The model under review builds one solid part; all positions refer to its coordinate system, in mm. Face numbers are marked on the shaded views. A direction names the side the tool comes from. Round coordinates to 2 decimals unless told otherwise and drop trailing zeros. Write each loop counter-clockwise with the first axis right and the second up, starting at its lowest first coordinate (ties: lowest second). Pieces come first, ordered by that corner, then holes. Notation, with made-up numbers: (38, 88) - (68, 88) arc R18 ccw to (68, 119) - close; hole circle Ø1 at (-17, 64.5). An arc over 180 degrees is marked (long way). Return JSON: item names as keys, results as strings.
from build123d import *

# Parameters (mm, degrees)
BOSS_EXTRUDE1_DEPTH = 40
SKETCH2_R           = 12.7
CUT_EXTRUDE2_DEPTH  = 40


with BuildPart() as part:
    # Sketch1 → Boss-Extrude1 (new body)
    with BuildSketch(Plane.XY):
        with BuildLine():
            Line((133.254134777, 0), (133.254134777, 8))
            Line((133.254134777, 8), (91.254134777, 8))
            ThreePointArc((91.254134777, 8), (33.254134777, 58.549124673), (-24.745865223, 8))
            Line((-24.745865223, 8), (-66.745865223, 8))
            Line((-66.745865223, 8), (-66.745865223, 0))
            Line((-66.745865223, 0), (-16.745865223, 0))
            ThreePointArc((-16.745865223, 0), (33.254134777, 50), (83.254134777, 0))
            Line((83.254134777, 0), (133.254134777, 0))
        make_face()
    extrude(amount=BOSS_EXTRUDE1_DEPTH)

    # Sketch2 → Cut-Extrude2 (cut)
    with BuildSketch(Plane(origin=(0, 8, 0), x_dir=(1, 0, 0), z_dir=(0, 1, 0))):
        with Locations(Location((-46.745865223, -20, 0), (0, 0, 180))):
            Circle(SKETCH2_R)
        with Locations(Location((113.254134777, -20, 0), (0, 0, 180))):
            Circle(SKETCH2_R)
    extrude(amount=-CUT_EXTRUDE2_DEPTH, mode=Mode.SUBTRACT)


solid = part.part
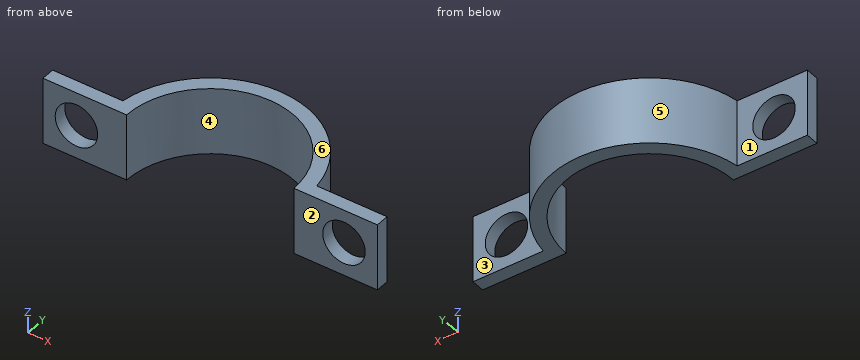
(1) Add section D-D (z = 9). Write out the cut boundary in (x, y), plus the area to 3 significant figures.
Filled in:
{"outline": "(-66.75, 0) - (-53.09, 0) - (-53.09, 8) - (-66.75, 8) - close; (-40.4, 0) - (-16.75, 0) arc R50 cw to (83.25, 0) - (106.91, 0) - (106.91, 8) - (91.25, 8) arc R58.55 ccw to (-24.75, 8) - (-40.4, 8) - close; (119.6, 0) - (133.25, 0) - (133.25, 8) - (119.6, 8) - close", "area": "1,920 mm2"}
(2) Add section B-B (y = 22.5). Write out the cut boundary in (x, z).
Filled in:
{"outline": "(-20.8, 0) - (-11.4, 0) - (-11.4, 40) - (-20.8, 40) - close; (77.91, 0) - (87.31, 0) - (87.31, 40) - (77.91, 40) - close"}
(3) Add section C-C (x = 103.5). Write out the cut boundary in (y, z), plus the area to 3 significant figures.
Filled in:
{"outline": "(0, 0) - (8, 0) - (8, 11.87) - (0, 11.87) - close; (0, 28.13) - (8, 28.13) - (8, 40) - (0, 40) - close", "area": "190 mm2"}
(4) Clearance check with flat-ended pins moving along their axes: pin 1 Ø5 at (y, z) = (21.5, 18) entering from +X; pin 2 Ø23 at (x, z) = (113.25, 20) entering from +Y; pin 3 Ø1.5 at (y, z) = (15, 35) entering from -X; pin 4 Ø20 at (x, z) = (-49, 10.5) entering from +Y. State where each tip first meets the part, or that it passes through.
Filled in:
{"pin 1": "stops at x = 88.63", "pin 2": "passes through", "pin 3": "stops at x = -23.53", "pin 4": "stops at y = 8"}
(5) For the marked faces 1, 2 and 3, list the 3-axis set-ups (+Z, -Z, +X, -X, +Y, -Y) from which the entire face can be reached by the end or side of a thin tool; tool diameter is ignored.
Filled in:
{"face 1": "+Z, -Z, -X, +Y", "face 2": "+Z, -Z, +X, -X, -Y", "face 3": "+Z, -Z, +X, +Y"}
(6) Mouldability with a two-part tool opening along X and no side actions: class the marked faces 4, 5 and 6 as released by +X, released by -X, zero draft, split by the parting line, or undercut.
Filled in:
{"face 4": "undercut", "face 5": "split by the parting line", "face 6": "zero draft"}
(7) Add section A-A (z = 20). Write out the cut boundary in (x, y), plus the area to 3 significant figures.
Filled in:
{"outline": "(-66.75, 0) - (-59.45, 0) - (-59.45, 8) - (-66.75, 8) - close; (-34.05, 0) - (-16.75, 0) arc R50 cw to (83.25, 0) - (100.55, 0) - (100.55, 8) - (91.25, 8) arc R58.55 ccw to (-24.75, 8) - (-34.05, 8) - close; (125.95, 0) - (133.25, 0) - (133.25, 8) - (125.95, 8) - close", "area": "1,720 mm2"}
(8) Wall thickness on line 1 (Y direction, x = 124, z = 7); line 2 (X direction, y = 26.5, z = 2); line 3 (X direction, y = 5, z = 27): over which ranges is each line inside the solid? List them lowest first.
Filled in:
{"line 1": "y = 0 to 8", "line 2": "x = -18.95 to -9.15, 75.65 to 85.46", "line 3": "x = -66.75 to -57.34, -36.15 to -16.5, 83 to 102.66, 123.85 to 133.25"}
